For this review, use the dimensioned drawing (mm, ordinates from the lowest corner) and the shaded views. A direction names the side the tool comes from. Round coordinates to 2 decimals unless told otherwise and drop trailing zeros. Write each loop counter-clockwise with the first axis right and the second up, starting at its lowest first coordinate (ties: lowest second). Pieces come first, ordered by that corner, then holes. Notation, with made-up numbers: (36, 79.5) - (40, 79.5) arc R31 ccw to (40, 109.5) - close; hole circle Ø4 at (85, 44). An arc over 180 degrees is marked (long way). Return JSON: item names as keys, results as strings.
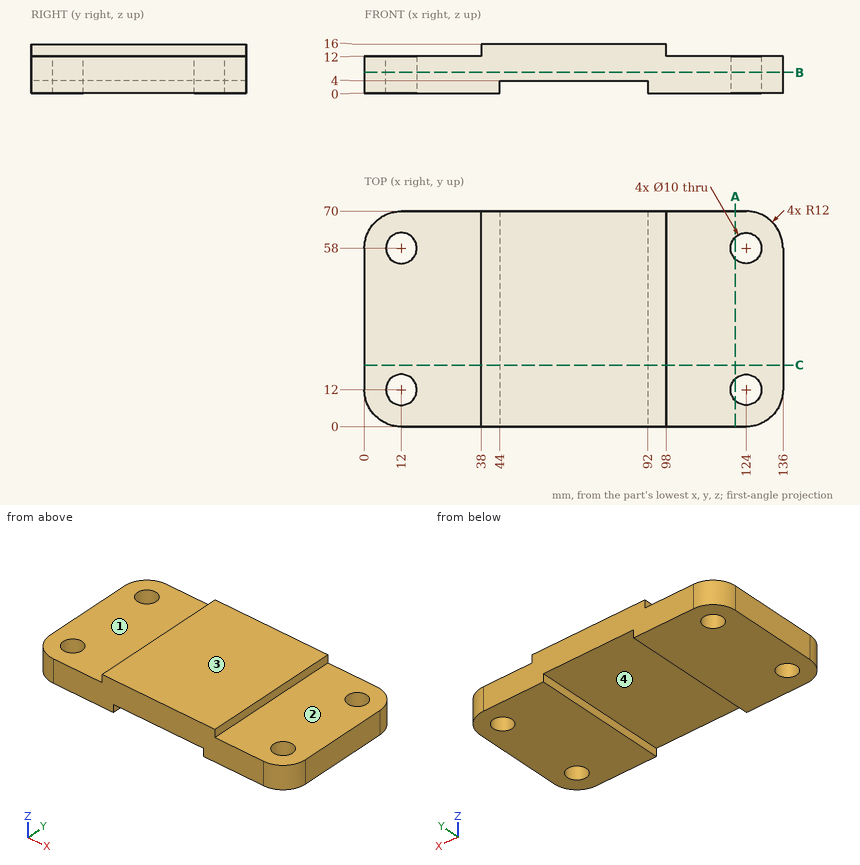
(1) Add section C-C (y = 20). Write out the cut boundary in (x, z).
Filled in:
{"outline": "(0, 0) - (44, 0) - (44, 4) - (92, 4) - (92, 0) - (136, 0) - (136, 12) - (98, 12) - (98, 16) - (38, 16) - (38, 12) - (0, 12) - close"}
(2) Clearance check with flat-ended pins moving along their axes: pin 1 Ø5 at (x, y) = (59, 38) entering from -Z; pin 2 Ø19 at (x, y) = (114.5, 25) entering from +Z; pin 3 Ø4.5 at (y, z) = (47.5, 15) entering from +X. State where each tip first meets the part, or that it passes through.
Filled in:
{"pin 1": "stops at z = 4", "pin 2": "stops at z = 12", "pin 3": "stops at x = 98"}
(3) Wall thickness on line 1 (Y direction, x = 124, z = 5.5); line 2 (X direction, y = 47.5, z = 3.5); line 3 (Y direction, x = 9.5, z = 3.25): over which ranges is each line inside the solid? List them lowest first.
Filled in:
{"line 1": "y = 0 to 7, 17 to 53, 63 to 70", "line 2": "x = 0 to 44, 92 to 136", "line 3": "y = 0.26 to 7.67, 16.33 to 53.67, 62.33 to 69.74"}
(4) Add section A-A (x = 120.5). Write out the cut boundary in (y, z).
Filled in:
{"outline": "(0, 0) - (8.43, 0) - (8.43, 12) - (0, 12) - close; (15.57, 0) - (54.43, 0) - (54.43, 12) - (15.57, 12) - close; (61.57, 0) - (70, 0) - (70, 12) - (61.57, 12) - close"}
(5) For the marked faces 1, 2, 3 and 4, list the 3-axis set-ups (+Z, -Z, +X, -X, +Y, -Y) from which the entire face can be reached by the end or side of a thin tool; tool diameter is ignored.
Filled in:
{"face 1": "+Z, -X, +Y, -Y", "face 2": "+Z, +X, +Y, -Y", "face 3": "+Z, +X, -X, +Y, -Y", "face 4": "-Z, +Y, -Y"}
(6) Add section B-B (z = 6.75). Write out the cut boundary in (x, y), plus the area to 3 significant figures.
Filled in:
{"outline": "(0, 12) arc R12 ccw to (12, 0) - (124, 0) arc R12 ccw to (136, 12) - (136, 58) arc R12 ccw to (124, 70) - (12, 70) arc R12 ccw to (0, 58) - close; hole circle Ø10 at (12, 12); hole circle Ø10 at (12, 58); hole circle Ø10 at (124, 12); hole circle Ø10 at (124, 58)", "area": "9,080 mm2"}
